Source: three-view drawing plus pictorial views. Frame: mm from the lowest corner of the part. Round coordinates to 2 decimals unless told otherwise and drop trailing zeros. Order: outer loops, then holes, each group sorted by start corner. A loop starts at its lowest first (then second) coordinate and runs counter-clockwise, first axis right, second up. Notation, with made-up numbers: (-29.75, -23) -> (12.25, -23) arc R24 ccw to (12.25, 15) -> close; hole circle Ø4 at (-15.75, 16.5). An arc over 180 degrees is marked (long way). Answer as CSV lines item,"result". Start each with the question number.
1) Section query C-C, the plane x = 100.5. Output: boundary loops of the cut face in (y, z).
2) Section query D-D, the plane y = 85.5. Output: boundary loops of the cut face in (x, z).
3) Section query B-B, the plane y = 56. Output: boundary loops of the cut face in (x, z).
4) Section query A-A, the plane x = 56. Output: boundary loops of the cut face in (y, z), and give its area (3 significant figures).
5) Line query: L1, parallel to Y at x = 56, z = 1.6; L2, parallel to Y at x = 87.5, z = 1.8 (1 decimal); L3, parallel to Y at x = 49.5, z = 0.8. Output: solid intervals per line, ascending.
6) First-contact query: P1, Ø22.5, axis at x = 56, y = 18.38, coming from the -Z side. Flat tip, straight axial feed; report the tip coordinate or a pass-through.
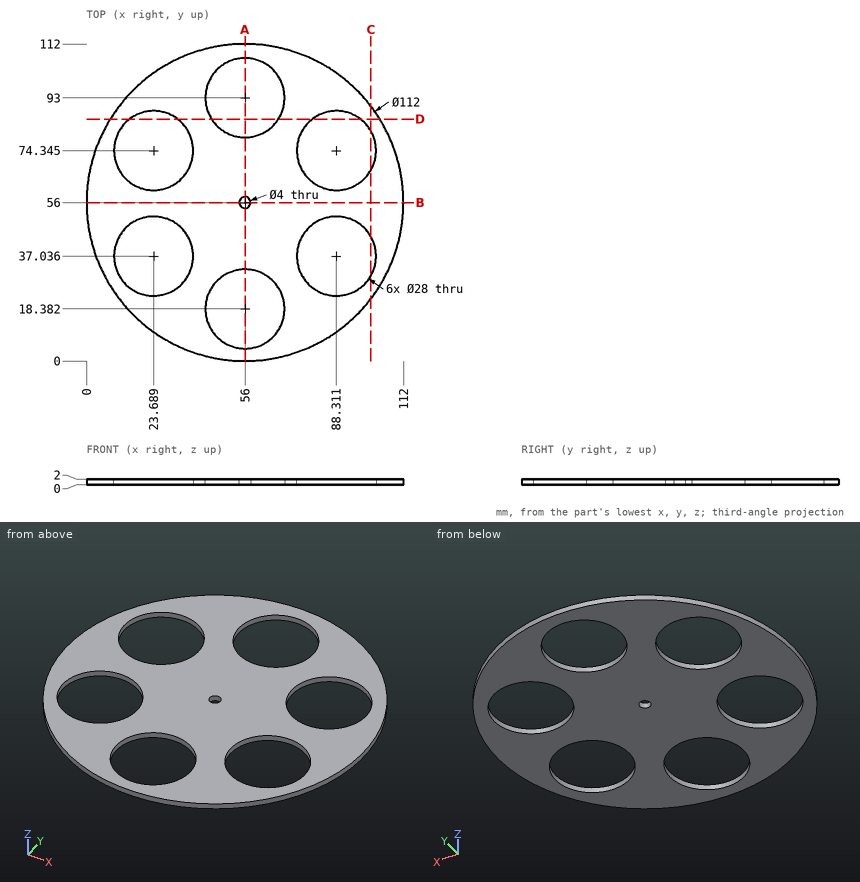
Findings:
1,outline,"(22, 0) -> (30.15, 0) -> (30.15, 2) -> (22, 2) -> close; (43.92, 0) -> (67.46, 0) -> (67.46, 2) -> (43.92, 2) -> close; (81.23, 0) -> (90, 0) -> (90, 2) -> (81.23, 2) -> close"
2,outline,"(8.4, 0) -> (15.23, 0) -> (15.23, 2) -> (8.4, 2) -> close; (32.15, 0) -> (44.18, 0) -> (44.18, 2) -> (32.15, 2) -> close; (67.82, 0) -> (79.85, 0) -> (79.85, 2) -> (67.82, 2) -> close; (96.77, 0) -> (103.6, 0) -> (103.6, 2) -> (96.77, 2) -> close"
3,outline,"(0, 0) -> (54, 0) -> (54, 2) -> (0, 2) -> close; (58, 0) -> (112, 0) -> (112, 2) -> (58, 2) -> close"
4,outline,"(0, 0) -> (4.38, 0) -> (4.38, 2) -> (0, 2) -> close; (32.38, 0) -> (54, 0) -> (54, 2) -> (32.38, 2) -> close; (58, 0) -> (79, 0) -> (79, 2) -> (58, 2) -> close; (107, 0) -> (112, 0) -> (112, 2) -> (107, 2) -> close"
4,area,"104 mm^2"
5,L1,"y = 0 to 4.38, 32.38 to 54, 58 to 79, 107 to 112"
5,L2,"y = 9.7 to 23.1, 51 to 60.4, 88.3 to 102.3"
5,L3,"y = 0.38 to 5.98, 30.78 to 80.6, 105.4 to 111.62"
6,P1,"passes through"
